```python
from build123d import *

# Parameters (mm, degrees)
F0_R     = 11
F1_DEPTH = 7
F2_R     = 1


# Not quite as in the source:
# - a feature names something its author has since deleted; it is built from what else it names


with BuildPart() as f1:
    # F0 (on Front) → F1 (new body)
    with BuildSketch(Plane.XZ):
        with BuildLine():
            ThreePointArc((14.5, 25.5), (0, 40), (-14.5, 25.5))
            Line((-14.5, 25.5), (-14.5, 8.3715789032))
            Line((-14.5, 8.3715789032), (-29.3336477965, -0.1926316451))
            ThreePointArc((-29.3336477965, -0.1926316451), (-34.6410161514, -20), (-14.8336477965, -25.3073683549))
            Line((-14.8336477965, -25.3073683549), (0, -16.7431578065))
            Line((0, -16.7431578065), (14.8336477965, -25.3073683549))
            ThreePointArc((14.8336477965, -25.3073683549), (34.6410161514, -20), (29.3336477965, -0.1926316451))
            Line((29.3336477965, -0.1926316451), (14.5, 8.3715789032))
            Line((14.5, 8.3715789032), (14.5, 25.5))
        make_face()
        with Locations((-22.0836477965, -12.75)):
            Circle(F0_R, mode=Mode.SUBTRACT)
        with BuildLine():
            ThreePointArc((-8.4021137105, -17.5526685347), (-7.7579062737, -14.9912339956), (-7.589017069, -12.355436857))
            ThreePointArc((-7.589017069, -12.355436857), (-5.2219051854, -13.5270730846), (-2.681534086, -14.2498903486))
            Line((-2.681534086, -14.2498903486), (-8.4021137105, -17.5526685347))
        make_face(mode=Mode.SUBTRACT)
        with BuildLine():
            ThreePointArc((-13.681534086, 4.8026685347), (-14.293919061, 2.4359552288), (-14.5, 0))
            ThreePointArc((-14.5, 0), (-14.4986576197, -0.1972998371), (-14.4946307275, -0.394563143))
            ThreePointArc((-14.4946307275, -0.394563143), (-16.8617426112, 0.7770730846), (-19.4021137105, 1.4998903486))
            Line((-19.4021137105, 1.4998903486), (-13.681534086, 4.8026685347))
        make_face(mode=Mode.SUBTRACT)
        with BuildLine():
            Line((8.4021137105, -17.5526685347), (2.681534086, -14.2498903486))
            ThreePointArc((2.681534086, -14.2498903486), (5.2219051854, -13.5270730846), (7.589017069, -12.355436857))
            ThreePointArc((7.589017069, -12.355436857), (7.7579062737, -14.9912339956), (8.4021137105, -17.5526685347))
        make_face(mode=Mode.SUBTRACT)
        with Locations((22.0836477965, -12.75)):
            Circle(F0_R, mode=Mode.SUBTRACT)
        Circle(F0_R, mode=Mode.SUBTRACT)
        with BuildLine():
            ThreePointArc((19.4021137105, 1.4998903486), (16.8617426112, 0.7770730846), (14.4946307275, -0.394563143))
            ThreePointArc((14.4946307275, -0.394563143), (14.4986576197, -0.1972998371), (14.5, 0))
            ThreePointArc((14.5, 0), (14.293919061, 2.4359552288), (13.681534086, 4.8026685347))
            Line((13.681534086, 4.8026685347), (19.4021137105, 1.4998903486))
        make_face(mode=Mode.SUBTRACT)
        with BuildLine():
            Line((-11, 9.4472218138), (-11, 16.0527781862))
            ThreePointArc((-11, 16.0527781862), (-9.1038363374, 14.214160911), (-6.9056136585, 12.75))
            ThreePointArc((-6.9056136585, 12.75), (-9.1038363374, 11.285839089), (-11, 9.4472218138))
        make_face(mode=Mode.SUBTRACT)
        with BuildLine():
            ThreePointArc((6.9056136585, 12.75), (9.1038363374, 14.214160911), (11, 16.0527781862))
            Line((11, 16.0527781862), (11, 9.4472218138))
            ThreePointArc((11, 9.4472218138), (9.1038363374, 11.285839089), (6.9056136585, 12.75))
        make_face(mode=Mode.SUBTRACT)
        with Locations((0, 25.5)):
            Circle(F0_R, mode=Mode.SUBTRACT)
    extrude(amount=F1_DEPTH)

    # F2
    f2_edges = [f1.edges().sort_by_distance(p)[0] for p in [
        (21.916824, -7, 4.089474),
        (14.5, -7, 16.935789),
        (14.5, 0, 16.935789),
        (21.916824, 0, 4.089474),
        (-7.416824, -7, -21.025263),
        (-21.916824, 0, 4.089474),
    ]]
    fillet(f2_edges, radius=F2_R)


solid = f1.part
```
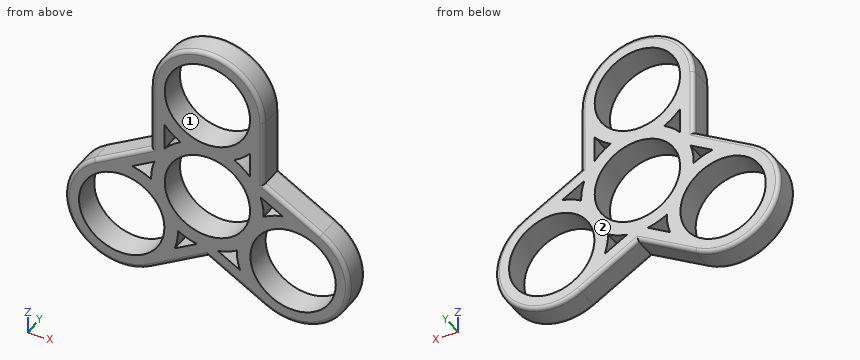
Input: part model. Units: mm. Frame: model coordinates. Face numbers are marked on the shaded views. Give positions to 0.01 mm unless a question says otherwise; leave off trailing zeros. One line per question, with ' | ' between items. Start each with the question number.
1. First-contact query: pin 1 Ø13 at (x, z) = (22.08, -12.75) entering from -Y; pin 2 Ø4 at (x, y) = (-3, -1.5) entering from -Z; pin 3 Ø2 at (y, z) = (-2.5, 12) entering from +X; pin 4 Ø2.5 at (y, z) = (-4.5, 16.5) entering from -X. Flat tips, straight axial feed; report the tip coordinate or a pass-through.
2. Pull-direction query (Z, two-part tool) for the marked faces 1 and 2; classes: released by +Z, released by -Z, zero draft, split by the parting line, or undercut.
3. Section query A-A (y = -5). Count the separate pieces of the cut face and the enclosed holes in it, and give its area (3 significant figures).
4. Material intervals for probe 1 along X at (y, z) = (-2.75, -22.5); probe 2 along Z at (x, y) = (-16.5, -0.75); probe 3 along Z at (x, y) = (2, -3.75), sorted ascending. Write a range as [from, to].
Here are the results:
1) pin 1: through | pin 2: z = -19.63 | pin 3: x = 14.5 | pin 4: x = -14.5
2) face 1: undercut | face 2: zero draft
3) separate pieces: 1 | enclosed holes: 10 | area: 1,250 mm²
4) probe 1: [-32.82, -27.18], [-16.99, -9.97], [9.97, 16.99], [27.18, 32.82] | probe 2: [-26.1, -22.23], [-3.27, 0.63], [3.18, 7.18] | probe 3: [-17.9, -10.82], [10.82, 14.68], [36.32, 39.86]
